The model under review builds one solid part; all positions refer to its coordinate system, in mm. A direction names the side the tool comes from. Round coordinates to 2 decimals unless told otherwise and drop trailing zeros. Order: outer loops, then holes, each group sorted by start corner. A loop starts at its lowest first (then second) coordinate and runs counter-clockwise, first axis right, second up. Notation, with made-up numbers: (7, -10) -> (22, -10) arc R25 cw to (22, 5) -> close; hole circle Ø2 at (-25, -14). An arc over 180 degrees is marked (long way). Use a Markdown table: item, result. Add a question column.
```python
from build123d import *

# Parameters (mm, degrees)
F0_W     = 1000
F0_H     = 1079.8176152468
F1_DEPTH = 1000
F2_R     = 40
F3_DEPTH = 1463.3684158325
F4_DEPTH = 25
F5_DEPTH = 334.466189146
F6_T     = -25
F7_R     = 10


with BuildPart() as f1:
    # F0 (on Front) → F1 (new body)
    with BuildSketch(Plane.XZ):
        with Locations((-87.0127184317, -2.3948438466)):
            Rectangle(F0_W, F0_H)
    extrude(amount=F1_DEPTH)

    # F2 (on face) → F3 (cut)
    with BuildSketch(Plane.XZ.offset(1000)):
        with Locations((-23.8594158151, 0)):
            Circle(F2_R)
    extrude(amount=-F3_DEPTH, mode=Mode.SUBTRACT)

    # F4 (add): a face of the model
    f4_faces = [f1.faces().sort_by_distance(p)[0] for p in [
        (-87.3080717633, -1000, -2.4060439751),
    ]]
    extrude(f4_faces, amount=F4_DEPTH)

    # F5 (add): a face of the model
    f5_faces = [f1.faces().sort_by_distance(p)[0] for p in [
        (-87.0127184317, -512.5, 537.5139637768),
    ]]
    extrude(f5_faces, amount=F5_DEPTH)

    # F6
    f6_openings = [f1.faces().sort_by_distance(p)[0] for p in [
        (-87.237974, -1025, 165.426197),
    ]]
    offset(amount=F6_T, openings=f6_openings)

    # F7
    f7_edges = [f1.edges().sort_by_distance(p)[0] for p in [
        (-88.859416, -25, 0),
    ]]
    fillet(f7_edges, radius=F7_R)


solid = f1.part
```
Q1. Add section A-A (y = -398). Write out the cut boundary in (x, z), then the cut area to 3 significant figures.
Q2. Add section C-C (x = 256.5). Write out the cut boundary in (y, z), then the cut area to 3 significant figures.
Q3. Add section D-D (z = 335.5). Write out the cut boundary in (x, y).
Q4. Machinability: for faces 4 (the flat face through (-587.013, -520, 155)), 5 (the flat face through (-562.013, -532, 155)), which of the approach directions +Z, -Z, +X, -X, +Y, -Y give a long, thin tool a straight path to every point of the face, cutting with its end or side? Answer none if there is none.
Q5. Mouldability with a two-part tool opening along X and no side actions: class faces 1 (the flat face through (412.987, -520, 155)), 2 (the flat face through (-89, -1025, -519)), 3 (the flat face through (387.987, -532, 155)) as pulls with the +X half, pulls with the -X half, needs draft (parallel to the pull), parting line crosses it, or undercut.
Q6. Add section B-B (z = 0). Write out the cut boundary in (x, y).
Q7. Wall thickness on line 1 (Z direction, x = -249, y = -758); line 2 (X direction, y = -787, z = -200.5); line 3 (Z direction, x = -35, y = -91): over which ranges is each line inside the solid? List them lowest first. Write a range as [from, to].
Q8. Insertion check: pin 1 (5 mm diameter, centred on x = -400.5, z = 82, fed in from +Y). The pin has a flat end and moves straight along its axis. Give the tip position at first contact, or say it passes through.
Report:
| question | item | result |
|---|---|---|
| 1 | outline | (-587.01, -542.3) -> (412.99, -542.3) -> (412.99, 871.98) -> (-587.01, 871.98) -> close; circle Ø130 at (-23.86, 0); hole (-562.01, -517.3) -> (387.99, -517.3) -> (387.99, 846.98) -> (-562.01, 846.98) -> close; hole circle Ø80 at (-23.86, 0) |
| 1 | area | 126,000 mm² |
| 2 | outline | (-1025, -542.3) -> (0, -542.3) -> (0, 871.98) -> (-1025, 871.98) -> (-1025, 846.98) -> (-25, 846.98) -> (-25, -517.3) -> (-1025, -517.3) -> close |
| 2 | area | 85,400 mm² |
| 3 | outline | (-587.01, -1025) -> (-562.01, -1025) -> (-562.01, -25) -> (387.99, -25) -> (387.99, -1025) -> (412.99, -1025) -> (412.99, 0) -> (-587.01, 0) -> close |
| 4 | face 4 | +Z, -Z, -X, +Y, -Y |
| 4 | face 5 | -Y |
| 5 | face 1 | pulls with the +X half |
| 5 | face 2 | needs draft |
| 5 | face 3 | undercut |
| 6 | outline | (-587.01, -1025) -> (-562.01, -1025) -> (-562.01, -25) -> (-98.86, -25) arc R10 cw to (-88.86, -35) -> (-88.86, -1025) -> (-63.86, -1025) -> (-63.86, 0) -> (-587.01, 0) -> close; (16.14, -1025) -> (41.14, -1025) -> (41.14, -35) arc R10 cw to (51.14, -25) -> (387.99, -25) -> (387.99, -1025) -> (412.99, -1025) -> (412.99, 0) -> (16.14, 0) -> close |
| 7 | line 1 | z = [-542.3, -517.3], [846.98, 871.98] |
| 7 | line 2 | x = [-587.01, -562.01], [387.99, 412.99] |
| 7 | line 3 | z = [-542.3, -517.3], [-64.04, -38.42], [38.42, 64.04], [846.98, 871.98] |
| 8 | pin 1 | stops at y = 0 |
